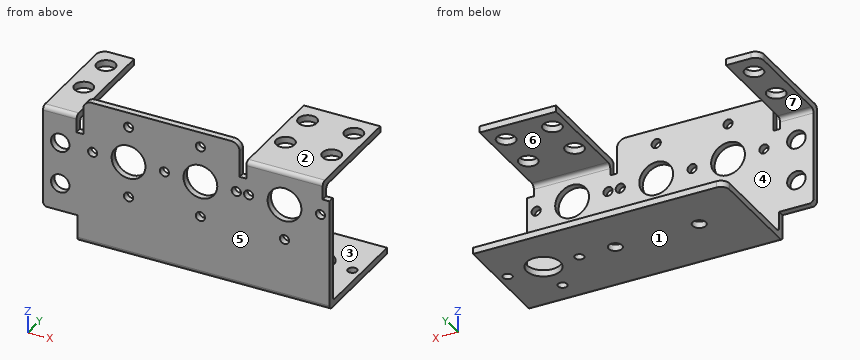
from build123d import *

# Parameters (mm, degrees)
SKETCH1_W                = 114.3
SKETCH1_H                = 34.72
BOSS_EXTRUDE1_DEPTH      = 1.524
SKETCH2_R                = 2.184
SKETCH2_W                = 8.15
SKETCH2_H                = 6.35
CUT_EXTRUDE1_DEPTH       = 1.524
SKETCH3_R                = 4
CUT_EXTRUDE2_DEPTH       = 50
SKETCH4_R                = 1.09
CUT_EXTRUDE3_DEPTH       = 50
CIRPATTERN1_COUNT        = 4
MIRROR2_COPY_1_SKETCH_R  = 1.09
MIRROR2_COPY_1_DEPTH     = 50
MIRROR2_COPY_2_SKETCH_R  = 1.09
MIRROR2_COPY_2_DEPTH     = 50
MIRROR2_COPY_3_SKETCH_R  = 1.09
MIRROR2_COPY_3_DEPTH     = 50
SKETCH7_R                = 4
CUT_EXTRUDE4_DEPTH       = 100
SKETCH8_R                = 1.09
CUT_EXTRUDE5_DEPTH       = 100
CIRPATTERN2_COUNT        = 4
SKETCH9_W                = 7.9375
SKETCH9_H                = 1.524
BOSS_EXTRUDE2_DEPTH      = 24.2
SKETCH10_W               = 98
SKETCH10_H               = 1.524
SKETCH10_W_2             = 18.075
BOSS_EXTRUDE3_DEPTH      = 24.2
SKETCH11_R               = 2.1844
CUT_EXTRUDE6_DEPTH       = 24.2
SKETCH12_R               = 2.1844
CUT_EXTRUDE8_DEPTH       = 24.2
FILLET1_R                = 1
SKETCH13_R               = 1.5875
CUT_EXTRUDE9_DEPTH       = 24.2
FILLET2_R                = 2
SKETCH14_R               = 4
CUT_EXTRUDE10_DEPTH      = 24.2
SKETCH15_R               = 1.09
CUT_EXTRUDE11_DEPTH      = 24.2
CIRPATTERN3_COUNT        = 4
CUT_EXTRUDE13_DEPTH      = 30
CUT_EXTRUDE13_DEPTH_BACK = 19
SKETCH18_W               = 48.234659097
SKETCH18_H               = 11.142394616
SKETCH18_H_2             = 30.082733934


with BuildPart() as part:
    # Sketch1 → Boss-Extrude1 (new body)
    with BuildSketch(Plane(origin=(0, 0, 0), x_dir=(1, 0, 0), z_dir=(0, 1, 0))):
        Rectangle(SKETCH1_W, SKETCH1_H)
    extrude(amount=BOSS_EXTRUDE1_DEPTH)

    # Sketch2 → Cut-Extrude1 (cut)
    with BuildSketch(Plane(origin=(0, 1.524, 0), x_dir=(1, 0, 0), z_dir=(0, 1, 0))):
        with Locations(Location((-53.075, 4.41, 0), (0, 0, 270))):
            Circle(SKETCH2_R)
        with Locations(Location((-53.075, -5.5, 0), (0, 0, 270))):
            Circle(SKETCH2_R)
        with Locations((-53.075, 14.185)):
            Rectangle(SKETCH2_W, SKETCH2_H)
        Polygon((-57.15, -13.36), (-49.2125, -13.36), (-49.2125, -9.16), (-47.625, -9.16), (-47.625, -13.36), (-47.625, -17.36), (-57.15, -17.36), align=None)
        Polygon((-10.625, -13.36), (-10.625, -9.16), (-9.0375, -9.16), (-9.0375, -13.36), (0, -13.36), (0, -17.36), (-10.625, -17.36), align=None)
    cut_extrude1 = extrude(amount=-CUT_EXTRUDE1_DEPTH, mode=Mode.SUBTRACT)

    # Mirror1: Cut-Extrude1 across plane
    add(cut_extrude1.mirror(Plane(origin=(0, 0, 0), x_dir=(0, 0, 1), z_dir=(1, 0, 0))), mode=Mode.SUBTRACT)

    # Sketch3 → Cut-Extrude2 (cut, symmetric)
    with BuildSketch(Plane(origin=(0, 1.524, 0), x_dir=(1, 0, 0), z_dir=(0, 1, 0))):
        with Locations(Location((-36.9062, -5.36, 0), (0, 0, 90))):
            Circle(SKETCH3_R)
    cut_extrude2 = extrude(amount=CUT_EXTRUDE2_DEPTH, both=True, mode=Mode.SUBTRACT)

    # Sketch4 → Cut-Extrude3 (cut, symmetric)
    with BuildSketch(Plane(origin=(0, 1.524, 0), x_dir=(1, 0, 0), z_dir=(0, 1, 0))):
        with Locations(Location((-36.9062, 3.14, 0), (0, 0, 90))):
            Circle(SKETCH4_R)
    cut_extrude3 = extrude(amount=CUT_EXTRUDE3_DEPTH, both=True, mode=Mode.SUBTRACT)

    # CirPattern1: Cut-Extrude3 ×4 about axis
    cirpattern1_axis = Axis((-36.9062, 0, 5.36), (0, 1, 0))
    for i in range(1, CIRPATTERN1_COUNT):
        add(cut_extrude3.rotate(cirpattern1_axis, i * 360 / CIRPATTERN1_COUNT), mode=Mode.SUBTRACT)

    # Mirror2: Cut-Extrude2, Cut-Extrude3 across plane
    add(cut_extrude2.mirror(Plane.ZY.offset(28.4062)), mode=Mode.SUBTRACT)
    add(cut_extrude3.mirror(Plane.ZY.offset(28.4062)), mode=Mode.SUBTRACT)

    # Mirror2 copy 1 sketch → Mirror2 copy 1 (cut, symmetric)
    with BuildSketch(Plane(origin=(-14.5462, 1.524, -31.5462), x_dir=(0, 0, -1), z_dir=(0, 1, 0))):
        with Locations((-36.9062, -3.14)):
            Circle(MIRROR2_COPY_1_SKETCH_R)
    extrude(amount=MIRROR2_COPY_1_DEPTH, both=True, mode=Mode.SUBTRACT)

    # Mirror2 copy 2 sketch → Mirror2 copy 2 (cut, symmetric)
    with BuildSketch(Plane(origin=(17, 1.524, 10.72), x_dir=(1, 0, 0), z_dir=(0, 1, 0))):
        with Locations((-36.9062, -3.14)):
            Circle(MIRROR2_COPY_2_SKETCH_R)
    extrude(amount=MIRROR2_COPY_2_DEPTH, both=True, mode=Mode.SUBTRACT)

    # Mirror2 copy 3 sketch → Mirror2 copy 3 (cut, symmetric)
    with BuildSketch(Plane(origin=(-25.2662, 1.524, 42.2662), x_dir=(0, 0, 1), z_dir=(0, 1, 0))):
        with Locations((-36.9062, -3.14)):
            Circle(MIRROR2_COPY_3_SKETCH_R)
    extrude(amount=MIRROR2_COPY_3_DEPTH, both=True, mode=Mode.SUBTRACT)

    # Sketch7 → Cut-Extrude4 (cut)
    with BuildSketch(Plane(origin=(0, 1.524, 0), x_dir=(1, 0, 0), z_dir=(0, 1, 0))):
        with Locations(Location((0, -5.36, 0), (0, 0, 270))):
            Circle(SKETCH7_R)
    extrude(amount=-CUT_EXTRUDE4_DEPTH, mode=Mode.SUBTRACT)

    # Sketch8 → Cut-Extrude5 (cut)
    with BuildSketch(Plane(origin=(0, 1.524, 0), x_dir=(1, 0, 0), z_dir=(0, 1, 0))):
        with Locations(Location((0, 3.14, 0), (0, 0, 270))):
            Circle(SKETCH8_R)
    cut_extrude5 = extrude(amount=-CUT_EXTRUDE5_DEPTH, mode=Mode.SUBTRACT)

    # CirPattern2: Cut-Extrude5 ×4 about axis, 1 skipped
    cirpattern2_axis = Axis((0, 0, 5.36), (0, 1, 0))
    add([cut_extrude5.rotate(cirpattern2_axis, i * 360 / CIRPATTERN2_COUNT) for i in range(1, CIRPATTERN2_COUNT) if i not in (2,)], mode=Mode.SUBTRACT)

    # Sketch9 → Boss-Extrude2 (add)
    with BuildSketch(Plane(origin=(0, 1.524, 0), x_dir=(1, 0, 0), z_dir=(0, 1, 0))):
        with Locations((-53.18125, -12.598)):
            Rectangle(SKETCH9_W, SKETCH9_H)
    boss_extrude2 = extrude(amount=BOSS_EXTRUDE2_DEPTH)

    # Mirror4: Boss-Extrude2 across plane
    add(boss_extrude2.mirror(Plane(origin=(0, 0, 0), x_dir=(0, 0, 1), z_dir=(1, 0, 0))))

    # Sketch10 → Boss-Extrude3 (add)
    with BuildSketch(Plane(origin=(0, 1.524, 0), x_dir=(1, 0, 0), z_dir=(0, 1, 0))):
        with Locations((0, 16.598)):
            Rectangle(SKETCH10_W, SKETCH10_H)
        with Locations((0, -12.598)):
            Rectangle(SKETCH10_W_2, SKETCH10_H)
    extrude(amount=BOSS_EXTRUDE3_DEPTH)

    # Sketch11 → Cut-Extrude6 (cut)
    with BuildSketch(Plane.XY.offset(13.36)):
        with Locations((-53.18125, 20.644)):
            Circle(SKETCH11_R)
        with Locations((-53.18125, 10.734)):
            Circle(SKETCH11_R)
    cut_extrude6 = extrude(amount=-CUT_EXTRUDE6_DEPTH, mode=Mode.SUBTRACT)

    # Mirror5: Cut-Extrude6 across plane
    add(cut_extrude6.mirror(Plane(origin=(0, 0, 0), x_dir=(0, 0, 1), z_dir=(1, 0, 0))), mode=Mode.SUBTRACT)

    # Sketch12 → Cut-Extrude8 (cut)
    with BuildSketch(Plane.XY.offset(13.36)):
        with Locations((-5.47125, 20.644)):
            Circle(SKETCH12_R)
        with Locations((-5.47125, 10.734)):
            Circle(SKETCH12_R)
        with Locations((5.47125, 10.734)):
            Circle(SKETCH12_R)
        with Locations((5.47125, 20.644)):
            Circle(SKETCH12_R)
    extrude(amount=-CUT_EXTRUDE8_DEPTH, mode=Mode.SUBTRACT)

    # Fillet1
    fillet1_edges = [part.edges().sort_by_distance(p)[0] for p in [
        (53.18125, 0, 13.36),
        (-53.18125, 1.524, 11.836),
        (53.18125, 1.524, 11.836),
        (0, 1.524, -15.836),
        (0, 1.524, 11.836),
        (-57.15, 0.762, -11.01),
        (-53.18125, 0, 13.36),
        (0, 0, 13.36),
        (0, 0, -17.36),
        (57.15, 0.762, -11.01),
    ]]
    fillet(fillet1_edges, radius=FILLET1_R)

    # Sketch13 → Cut-Extrude9 (cut)
    with BuildSketch(Plane.XY.offset(-15.836)):
        with Locations((36.8628, 14.2875)):
            Circle(SKETCH13_R)
        with Locations((17, 14.2875)):
            Circle(SKETCH13_R)
    cut_extrude9 = extrude(amount=-CUT_EXTRUDE9_DEPTH, mode=Mode.SUBTRACT)

    # Mirror6: Cut-Extrude9 across plane
    add(cut_extrude9.mirror(Plane(origin=(0, 0, 0), x_dir=(0, 0, 1), z_dir=(1, 0, 0))), mode=Mode.SUBTRACT)

    # Fillet2
    fillet2_edges = [part.edges().sort_by_distance(p)[0] for p in [
        (47.625, 0.762, 17.36),
        (10.625, 0.762, 17.36),
        (-57.15, 25.724, 12.598),
        (57.15, 25.724, 12.598),
        (-49, 25.724, -16.598),
        (49, 25.724, -16.598),
        (-47.625, 0.762, 17.36),
        (-10.625, 0.762, 17.36),
    ]]
    fillet(fillet2_edges, radius=FILLET2_R)

    # Sketch14 → Cut-Extrude10 (cut)
    with BuildSketch(Plane.XY.offset(-15.836)):
        with Locations((0, 14.2875)):
            Circle(SKETCH14_R)
    extrude(amount=-CUT_EXTRUDE10_DEPTH, mode=Mode.SUBTRACT)

    # Sketch15 → Cut-Extrude11 (cut)
    with BuildSketch(Plane.XY.offset(-15.836)):
        with Locations((0, 5.7875)):
            Circle(SKETCH15_R)
    cut_extrude11 = extrude(amount=-CUT_EXTRUDE11_DEPTH, mode=Mode.SUBTRACT)

    # CirPattern3: Cut-Extrude11 ×4 about axis, 1 skipped
    cirpattern3_axis = Axis((0, 14.2875, 0), (0, 0, 1))
    add([cut_extrude11.rotate(cirpattern3_axis, i * 360 / CIRPATTERN3_COUNT) for i in range(1, CIRPATTERN3_COUNT) if i not in (2,)], mode=Mode.SUBTRACT)

    # Sketch18 → Cut-Extrude13 (cut, two sides: drawn at the far end of the back side and taken through both)
    with BuildSketch(Plane(origin=(0, 1.524, 0), x_dir=(1, 0, 0), z_dir=(0, 1, 0)).offset(-CUT_EXTRUDE13_DEPTH_BACK)):
        with Locations((34.742329549, -14.731197308)):
            Rectangle(SKETCH18_W, SKETCH18_H)
        with Locations((34.742329549, 5.881366967)):
            Rectangle(SKETCH18_W, SKETCH18_H_2)
    extrude(amount=CUT_EXTRUDE13_DEPTH + CUT_EXTRUDE13_DEPTH_BACK, mode=Mode.SUBTRACT)


solid = part.part
Design review of the part built by this model. Coordinates are the model's own, in mm. Face numbers are marked on the shaded views. A direction names the side the tool comes from. Round coordinates to 2 decimals unless told otherwise and drop trailing zeros. Write each loop counter-clockwise with the first axis right and the second up, starting at its lowest first coordinate (ties: lowest second). Pieces come first, ordered by that corner, then holes. Notation, with made-up numbers: (19.5, -38) -> (68.5, -38) arc R28 cw to (68.5, -13) -> close; hole circle Ø7 at (27, 72.25). An arc over 180 degrees is marked (long way). One line per question, with ' | ' between items.
(1) Take a section at A-A, the plane x = 0. State the section outline as (y, z) points, and give its area (4 significant figures).
Result sheet:
outline: (0, -16.36) arc R1 ccw to (1, -17.36) -> (4.7, -17.36) -> (4.7, -15.84) -> (2.52, -15.84) arc R1 cw to (1.52, -14.84) -> (1.52, -4.23) -> (0, -4.23) -> close; (0, -2.05) -> (1.52, -2.05) -> (1.52, 1.36) -> (0, 1.36) -> close; (0, 9.36) -> (1.52, 9.36) -> (1.52, 10.84) arc R1 cw to (2.52, 11.84) -> (25.72, 11.84) -> (25.72, 13.36) -> (1, 13.36) arc R1 ccw to (0, 12.36) -> close; (6.88, -17.36) -> (10.29, -17.36) -> (10.29, -15.84) -> (6.88, -15.84) -> close; (18.29, -17.36) -> (25.72, -17.36) -> (25.72, -15.84) -> (18.29, -15.84) -> close | area: 89.55 mm2
(2) Take a section at B-B, the plane x = -22. State the section outline as (y, z) points, and give its area (3 significant figures).
Result sheet:
outline: (0, -16.36) arc R1 ccw to (1, -17.36) -> (25.72, -17.36) -> (25.72, -15.84) -> (2.52, -15.84) arc R1 cw to (1.52, -14.84) -> (1.52, 1.95) -> (0, 1.95) -> close; (0, 8.77) -> (1.52, 8.77) -> (1.52, 17.36) -> (0, 17.36) -> close | area: 79.4 mm2
(3) Draft analysis for pull direction Z (two halves, no side actions). For the marked faces 1, 2, 3 and 4, state which applies: released by +Z, released by -Z, zero draft, split by the parting line, or undercut.
Result sheet:
face 1: released by -Z | face 2: released by +Z | face 3: undercut | face 4: undercut
(4) Wall thickness on line 1 (Z direction, x = 4, y = 8.75); line 2 (Y direction, x = -26.5, z = -6); line 3 (Z direction, x = 5, y = 20): over which ranges is each line inside the solid? List them lowest first. Write a range as [from, to].
Result sheet:
line 1: [-17.36, -15.84], [11.84, 13.36] | line 2: [0, 1.52] | line 3: [-17.36, -15.84]
(5) Insertion check: P1, Ø1.9, axis at x = -17, y = 14.29, coming from the +Z side; P2, Ø0.5, axis at x = 9.5, y = 0.5, coming from the +Z side; P3, Ø2, axis at x = -32.5, y = 20.5, coming from the +Z side; P4, Ø5, axis at x = -53.075, z = 5.5, coming from the +Y side. Each pin has a flat end and moves straight along its axis. Give the tip position at first contact, or say it passes through.
Result sheet:
P1: through | P2: z = 9.16 | P3: z = -15.84 | P4: y = 1.52
(6) Take a section at C-C, the plane z = 5.36. State how many separate pieces and enclosed holes the cut face has, and give its area (3 significant figures).
Result sheet:
separate pieces: 10 | enclosed holes: 0 | area: 43.5 mm2
(7) Machinability: for the marked faces 5, 6 and 7, which of the approach directions +Z, -Z, +X, -X, +Y, -Y give a long, thin tool a straight path to every point of the face, cutting with its end or side? Answer none if there is none.
Result sheet:
face 5: +Z, -Z, +X, -X, -Y | face 6: +X, -X, +Y | face 7: -Z, +X, -X, +Y
